Autodesk Inventor part; units mm, degrees
ref_plane "YZ Plane" through (0, 0, 0) normal (1, 0, 0) x (0, 1, 0)
ref_plane "XZ Plane" through (0, 0, 0) normal (0, 1, 0) x (-1, 0, 0)
ref_plane "XY Plane" through (0, 0, 0) normal (0, 0, 1) x (1, 0, 0)
sketch "Sketch_40" plane through (0, 0, 0) normal (0, 0, 1) x (1, 0, 0)
  line L0 (3, 0) -> (-3, 0)
  line L1 (0, 5.175) -> (0, 4.3)
  arc A0 (0, 4.3) -> (0.3, 4) centre (0.3, 4.3) ccw
  line L2 (0.3, 4) -> (5.7, 4)
  arc A1 (5.7, 4) -> (6, 4.3) centre (5.7, 4.3) ccw
  line L3 (6, 4.3) -> (6, 5.175)
  arc A2 (6, 5.175) -> (5.925, 5.25) centre (5.925, 5.175) ccw
  line L4 (5.925, 5.25) -> (3.9786, 5.25)
  arc A3 (2.0214, 5.25) -> (3.9786, 5.25) centre (3, 6.5) ccw
  line L5 (2.0214, 5.25) -> (0.075, 5.25)
  arc A4 (0.075, 5.25) -> (0, 5.175) centre (0.075, 5.175) ccw
revolve "Revolution1" add sketch "Sketch_40" angle 360 about axis through (3, 0, 0) along (1, 0, 0)
sketch "Sketch_42" plane through (0, 0, 0) normal (0, 0, 1) x (1, 0, 0)
  line L0 (3, 0) -> (-3, 0)
  line L1 (0, 11.4) -> (0, 4.9)
  line L2 (0, 4.9) -> (0.15, 4.9)
  arc A0 (0.15, 4.9) -> (0.45, 5.2) centre (0.15, 5.2) ccw
  line L3 (0.45, 5.2) -> (0.45, 11.1)
  line L4 (0.45, 11.1) -> (5.55, 11.1)
  line L5 (5.55, 11.1) -> (5.55, 5.2)
  arc A1 (5.55, 5.2) -> (5.85, 4.9) centre (5.85, 5.2) ccw
  line L6 (5.85, 4.9) -> (6, 4.9)
  line L7 (6, 4.9) -> (6, 11.4)
  line L8 (6, 11.4) -> (0, 11.4)
revolve "Revolution2" cut sketch "Sketch_42" angle 360 about axis through (3, 0, 0) along (1, 0, 0)
sketch "Sketch_43" plane through (0, 0, 0) normal (0, 0, 1) x (1, 0, 0)
  line L0 (50, 0) -> (-50, 0)
  line L1 (0.075, 7.75) -> (0.12, 7.0375)
  line L2 (0.12, 7.0375) -> (0.075, 6.325)
  line L3 (0.075, 6.325) -> (0.075, 4.9)
  line L4 (0.075, 4.9) -> (0.165, 4.9)
  line L5 (0.165, 4.9) -> (0.255, 6.325)
  line L6 (0.255, 6.325) -> (0.255, 7.0375)
  line L7 (0.255, 7.0375) -> (0.165, 7.75)
  line L8 (0.165, 7.75) -> (0.075, 7.75)
revolve "Revolution3" add sketch "Sketch_43" angle 360 about axis through (50, 0, 0) along (1, 0, 0)
sketch "Sketch_44" plane through (0, 0, 0) normal (0, 0, 1) x (1, 0, 0)
  line L0 (50, 0) -> (-50, 0)
  line L1 (5.745, 7.0375) -> (5.745, 6.325)
  line L2 (5.745, 6.325) -> (5.835, 4.9)
  line L3 (5.835, 4.9) -> (5.925, 4.9)
  line L4 (5.925, 4.9) -> (5.925, 6.325)
  line L5 (5.925, 6.325) -> (5.88, 7.0375)
  line L6 (5.88, 7.0375) -> (5.925, 7.75)
  line L7 (5.925, 7.75) -> (5.835, 7.75)
  line L8 (5.835, 7.75) -> (5.745, 7.0375)
revolve "Revolution4" add sketch "Sketch_44" angle 360 about axis through (50, 0, 0) along (1, 0, 0)
properties part number "W 619/8 R-2Z_PART1"
Geometry check sheet. Reference: the model listing, model coordinates, mm. A direction names the side the tool comes from. Coordinates: 2 decimals unless noted, no trailing zeros. Loops run counter-clockwise (first coordinate to the right, second up) from the corner with the lowest first, then second, coordinate; pieces in that order, holes last. Notation, with made-up numbers: (84, 45) - (93, 45) arc R10 cw to (93, 53) - close; hole circle Ø7 at (46, 0). An arc over 180 degrees is marked (long way). Use one line per item in the form item = value. Start each with the question number.
Item 1: Section check B-B, the plane x = 2.65. Enter the section's corners in (y, z), and give its area (3 significant figures).
Item 2: Mould release check, pull along Y, two halves, no side actions. Record for faces 1 (the face through (3.038, -0.867, -3.905)), 2 (the face through (0, 2, -4)), 3 (the face through (4.8, 5, -1.6)): +Y half, -Y half, draft (parallel to the pull), parting line (faces both ways), or undercut.
Item 3: Thickness scan on probe 1 along Z at (x, y) = (1.5, 0); probe 2 along X at (y, z) = (3, -5.5) (3 decimals); probe 3 along Z at (x, y) = (2.95, 0). Record the ranges inside material, lowest first.
Item 4: Gauge pin test, flat ends, axial feed: pin 1 (3 mm diameter, centred on y = 0.5, z = 0, fed in from +X); pin 2 (6.5 mm diameter, centred on y = -2, z = -2, fed in from +X); pin 3 (1 mm diameter, centred on x = 4, y = -2, fed in from +Z); pin 4 (1.5 mm diameter, centred on x = 1.5, y = 5, fed in from -Z). Record the tip position at first contact, or that the pin passes through.
Item 5: Tool access check on faces 4 (the face through (6, 2, -4)), 5 (the face through (0.255, -6, 3)). Record the directions out of +Z, -Z, +X, -X, +Y, -Y that give a thin tool (end or side, any length) a straight path to the whole face; none if there is none.
Item 6: Section check A-A, the plane x = 1.4. Enter the section's corners in (y, z).
Computed:
q1.outline = circle Ø9.9 at (0, 0); hole circle Ø8 at (0, 0)
q1.area = 26.8 mm2
q2.face_1 = undercut
q2.face_2 = draft
q2.face_3 = parting line
q3.probe_1 = -5.25 to -4, 4 to 5.25
q3.probe_2 = 0.075 to 0.251, 5.749 to 5.925
q3.probe_3 = -4.91 to -4, 4 to 4.91
q4.pin_1 = through
q4.pin_2 = 6
q4.pin_3 = 5.03
q4.pin_4 = -3.08
q5.face_4 = +Z, -Z, +X, +Y, -Y
q5.face_5 = none
q6.outline = circle Ø10.5 at (0, 0); hole circle Ø8 at (0, 0)
